Model file for the job. Use its own axes, mm. A direction names the side the tool comes from. Round coordinates to 2 decimals unless told otherwise and drop trailing zeros. Order: outer loops, then holes, each group sorted by start corner. A loop starts at its lowest first (then second) coordinate and runs counter-clockwise, first axis right, second up. Notation, with made-up numbers: (65.5, 76.5) -> (104.5, 76.5) arc R32 cw to (104.5, 105.5) -> close; hole circle Ø1 at (-38.5, 16.25). An arc over 180 degrees is marked (long way). Answer as CSV lines item,"result".
```python
from build123d import *

# Parameters (mm, degrees)
F0_R     = 7.5
F1_DEPTH = 20
F2_DEPTH = 35
F3_R     = 15
F4_DEPTH = 25
F5_R     = 3.175
F6_DEPTH = 31.5


with BuildPart() as f1:
    # F0 (on Top) → F1 (new body)
    with BuildSketch(Plane.XY):
        with BuildLine():
            Line((0, 40), (0, 50))
            ThreePointArc((0, 50), (-5.8547207654, 49.6560393584), (-11.6288897904, 48.6288897904))
            Line((-11.6288897904, 48.6288897904), (-5, 42))
            Line((-5, 42), (-15, 42))
            Line((-15, 42), (-15, 47.6969600708))
            ThreePointArc((-15, 47.6969600708), (-17.5249921621, 46.8281395073), (-20, 45.8257569496))
            Line((-20, 45.8257569496), (-20, -20))
            Line((-20, -20), (0, -20))
            Line((0, -20), (43.72135955, -20))
            Line((43.72135955, -20), (44.72135955, -20))
            Line((44.72135955, -20), (44.72135955, 1))
            ThreePointArc((44.72135955, 1), (44.4284663312, 0.2928932188), (43.72135955, 0))
            Line((43.72135955, 0), (40, 0))
            ThreePointArc((40, 0), (11.7157287525, 11.7157287525), (0, 40))
        make_face()
        with Locations((-10, -10)):
            Circle(F0_R, mode=Mode.SUBTRACT)
        Polygon((8, -5), (18, -5), (8, -15), align=None, mode=Mode.SUBTRACT)
        Polygon((35, -15), (25, -15), (35, -5), align=None, mode=Mode.SUBTRACT)
        Polygon((-15, 8), (-15, 18), (-5, 8), align=None, mode=Mode.SUBTRACT)
        Polygon((-5, 35), (-5, 25), (-15, 35), align=None, mode=Mode.SUBTRACT)
        with BuildLine():
            Line((0, 50), (0, 60))
            ThreePointArc((0, 60), (-10.1461187235, 59.1359135792), (-20, 56.5685424949))
            Line((-20, 56.5685424949), (-20, 45.8257569496))
            ThreePointArc((-20, 45.8257569496), (-17.5249921621, 46.8281395073), (-15, 47.6969600708))
            Line((-15, 47.6969600708), (-15, 52))
            Line((-15, 52), (-11.6288897904, 48.6288897904))
            ThreePointArc((-11.6288897904, 48.6288897904), (-5.8547207654, 49.6560393584), (0, 50))
        make_face()
        with BuildLine():
            Line((0, 60), (0, 70))
            ThreePointArc((0, 70), (-2.5032041292, 69.9552283185), (-5.0032061825, 69.8209705454))
            ThreePointArc((-5.0032061825, 69.8209705454), (-9.2928932188, 65.0502525317), (-14.7467938175, 68.4290294546))
            ThreePointArc((-14.7467938175, 68.4290294546), (-17.3864463232, 67.8064265704), (-20, 67.082039325))
            Line((-20, 67.082039325), (-20, 56.5685424949))
            ThreePointArc((-20, 56.5685424949), (-10.1461187235, 59.1359135792), (0, 60))
        make_face()
        with BuildLine():
            Line((0, 70), (0, 80))
            ThreePointArc((0, 80), (-10.0803433986, 79.3623757014), (-20, 77.4596669241))
            Line((-20, 77.4596669241), (-20, 67.082039325))
            ThreePointArc((-20, 67.082039325), (-17.3864463232, 67.8064265704), (-14.7467938175, 68.4290294546))
            ThreePointArc((-14.7467938175, 68.4290294546), (-10.7956226846, 74.936292591), (-5, 70))
            ThreePointArc((-5, 70), (-5.0008016099, 69.9104709192), (-5.0032061825, 69.8209705454))
            ThreePointArc((-5.0032061825, 69.8209705454), (-2.5032041292, 69.9552283185), (0, 70))
        make_face()
        with BuildLine():
            ThreePointArc((-20, 77.4596669241), (-10.0803433986, 79.3623757014), (0, 80))
            Line((0, 80), (-20, 80))
            Line((-20, 80), (-20, 77.4596669241))
        make_face()
        with BuildLine():
            ThreePointArc((50, 0), (48.6624494734, 11.4876460274), (44.72135955, 22.360679775))
            Line((44.72135955, 22.360679775), (44.72135955, 1))
            Line((44.72135955, 1), (44.72135955, -20))
            Line((44.72135955, -20), (44.72135955, -21))
            Line((44.72135955, -21), (44.72135955, -22.360679775))
            ThreePointArc((44.72135955, -22.360679775), (48.6624494734, -11.4876460274), (50, 0))
        make_face()
        with BuildLine():
            ThreePointArc((60, 0), (56.0503415378, 21.4093253864), (44.72135955, 40))
            Line((44.72135955, 40), (44.72135955, 22.360679775))
            ThreePointArc((44.72135955, 22.360679775), (48.6624494734, 11.4876460274), (50, 0))
            ThreePointArc((50, 0), (48.6624494734, -11.4876460274), (44.72135955, -22.360679775))
            Line((44.72135955, -22.360679775), (44.72135955, -40))
            ThreePointArc((44.72135955, -40), (56.0503415378, -21.4093253864), (60, 0))
        make_face()
        with BuildLine():
            ThreePointArc((70, 0), (66.7877004117, 20.9619434622), (57.4456264654, 40))
            Line((57.4456264654, 40), (44.72135955, 40))
            ThreePointArc((44.72135955, 40), (56.0503415378, 21.4093253864), (60, 0))
            ThreePointArc((60, 0), (56.0503415378, -21.4093253864), (44.72135955, -40))
            Line((44.72135955, -40), (57.4456264654, -40))
            ThreePointArc((57.4456264654, -40), (66.7877004117, -20.9619434622), (70, 0))
        make_face()
        with BuildLine():
            ThreePointArc((79.72135955, 6.6711941585), (76.3426815131, 23.9122349309), (69.2820323028, 40))
            Line((69.2820323028, 40), (57.4456264654, 40))
            ThreePointArc((57.4456264654, 40), (66.7877004117, 20.9619434622), (70, 0))
            ThreePointArc((70, 0), (66.7877004117, -20.9619434622), (57.4456264654, -40))
            Line((57.4456264654, -40), (69.2820323028, -40))
            ThreePointArc((69.2820323028, -40), (76.3426815131, -23.9122349309), (79.72135955, -6.6711941585))
            Line((79.72135955, -6.6711941585), (79.72135955, 6.6711941585))
        make_face()
        with BuildLine():
            ThreePointArc((69.2820323028, 40), (40, 69.2820323028), (0, 80))
            Line((0, 80), (0, 70))
            ThreePointArc((0, 70), (32.403703492, 62.04836823), (57.4456264654, 40))
            Line((57.4456264654, 40), (69.2820323028, 40))
        make_face()
        with BuildLine():
            ThreePointArc((44.72135955, 40), (24.4948974278, 54.7722557505), (0, 60))
            Line((0, 60), (0, 50))
            ThreePointArc((0, 50), (26.286555606, 42.5325404176), (44.72135955, 22.360679775))
            Line((44.72135955, 22.360679775), (44.72135955, 40))
        make_face()
        with BuildLine():
            Line((79.72135955, 40), (69.2820323028, 40))
            ThreePointArc((69.2820323028, 40), (76.3426815131, 23.9122349309), (79.72135955, 6.6711941585))
            Line((79.72135955, 6.6711941585), (79.72135955, 40))
        make_face()
        with BuildLine():
            ThreePointArc((79.72135955, -6.6711941585), (76.3426815131, -23.9122349309), (69.2820323028, -40))
            Line((69.2820323028, -40), (79.72135955, -40))
            Line((79.72135955, -40), (79.72135955, -6.6711941585))
        make_face()
    extrude(amount=F1_DEPTH)

    # F0 (on Top) → F2 (join)
    with BuildSketch(Plane.XY):
        with BuildLine():
            ThreePointArc((50, 0), (48.6624494734, 11.4876460274), (44.72135955, 22.360679775))
            Line((44.72135955, 22.360679775), (44.72135955, 1))
            Line((44.72135955, 1), (44.72135955, -20))
            Line((44.72135955, -20), (44.72135955, -21))
            Line((44.72135955, -21), (44.72135955, -22.360679775))
            ThreePointArc((44.72135955, -22.360679775), (48.6624494734, -11.4876460274), (50, 0))
        make_face()
        with BuildLine():
            ThreePointArc((60, 0), (56.0503415378, 21.4093253864), (44.72135955, 40))
            Line((44.72135955, 40), (44.72135955, 22.360679775))
            ThreePointArc((44.72135955, 22.360679775), (48.6624494734, 11.4876460274), (50, 0))
            ThreePointArc((50, 0), (48.6624494734, -11.4876460274), (44.72135955, -22.360679775))
            Line((44.72135955, -22.360679775), (44.72135955, -40))
            ThreePointArc((44.72135955, -40), (56.0503415378, -21.4093253864), (60, 0))
        make_face()
        with BuildLine():
            ThreePointArc((70, 0), (66.7877004117, 20.9619434622), (57.4456264654, 40))
            Line((57.4456264654, 40), (44.72135955, 40))
            ThreePointArc((44.72135955, 40), (56.0503415378, 21.4093253864), (60, 0))
            ThreePointArc((60, 0), (56.0503415378, -21.4093253864), (44.72135955, -40))
            Line((44.72135955, -40), (57.4456264654, -40))
            ThreePointArc((57.4456264654, -40), (66.7877004117, -20.9619434622), (70, 0))
        make_face()
        with BuildLine():
            ThreePointArc((79.72135955, 6.6711941585), (76.3426815131, 23.9122349309), (69.2820323028, 40))
            Line((69.2820323028, 40), (57.4456264654, 40))
            ThreePointArc((57.4456264654, 40), (66.7877004117, 20.9619434622), (70, 0))
            ThreePointArc((70, 0), (66.7877004117, -20.9619434622), (57.4456264654, -40))
            Line((57.4456264654, -40), (69.2820323028, -40))
            ThreePointArc((69.2820323028, -40), (76.3426815131, -23.9122349309), (79.72135955, -6.6711941585))
            Line((79.72135955, -6.6711941585), (79.72135955, 6.6711941585))
        make_face()
        with BuildLine():
            ThreePointArc((79.72135955, -6.6711941585), (76.3426815131, -23.9122349309), (69.2820323028, -40))
            Line((69.2820323028, -40), (79.72135955, -40))
            Line((79.72135955, -40), (79.72135955, -6.6711941585))
        make_face()
        with BuildLine():
            Line((79.72135955, 40), (69.2820323028, 40))
            ThreePointArc((69.2820323028, 40), (76.3426815131, 23.9122349309), (79.72135955, 6.6711941585))
            Line((79.72135955, 6.6711941585), (79.72135955, 40))
        make_face()
    extrude(amount=F2_DEPTH)

    # F3 (on face) → F4 (cut)
    with BuildSketch(Plane.YZ.offset(79.72135955)):
        with Locations((0, 17.5)):
            Circle(F3_R)
    extrude(amount=-F4_DEPTH, mode=Mode.SUBTRACT)

    # F5 (on face) → F6 (cut)
    with BuildSketch(Plane.XY.offset(35)):
        with Locations((72.72135955, 0)):
            Circle(F5_R)
    extrude(amount=-F6_DEPTH, mode=Mode.SUBTRACT)


solid = f1.part
```
Q1. Saw through at C-C (z = 30.5). Write the cut outline in (x, y).
Checks:
outline,"(44.72, -40) -> (79.72, -40) -> (79.72, -7.48) -> (54.72, -7.48) -> (54.72, 7.48) -> (79.72, 7.48) -> (79.72, 40) -> (44.72, 40) -> close"
Q2. Mould opens along X. For faces 4 (the flat face through (12, -20, 10)), 5 (the flat face through (-20, 31, 10)), 6 (the flat face through (0, 45, 10)) say: +X half, -X half, draft (parallel to the pull), parting line (faces both ways), or undercut.
Checks:
face 4,"draft"
face 5,"-X half"
face 6,"undercut"
Q3. Wall check: L1, parallel to Y at x = 71, z = 17; L2, parallel to Y at x = 3, z = 9; L3, parallel to X at y = 30, z = 7. Give the ranges that are in metal, low to high. Write a range as [from, to].
Checks:
L1,"[-40, -14.99], [14.99, 40]"
L2,"[-20, 24.8], [49.91, 59.92], [69.94, 79.94]"
L3,"[-20, -10], [-5, 1.27], [40, 79.72]"
Q4. Flat gauge pins, fed straight in: pin 1 (12 mm diameter, centred on x = 1.5, y = 47, fed in from -Z); pin 2 (4 mm diameter, centred on x = 5.5, z = 8, fed in from +Y); pin 3 (10 mm diameter, centred on x = 20, z = 7.5, fed in from -Y); pin 4 (3 mm diameter, centred on x = 28.5, z = 11.5, fed in from +Y). Where does each tip first touch, or does it go through?
Checks:
pin 1,"z = 0"
pin 2,"y = 79.92"
pin 3,"y = -20"
pin 4,"y = 75.31"
Q5. Saw through at A-A (x = -10). Write the cut outline in (y, z).
Checks:
outline,"(-20, 0) -> (-17.5, 0) -> (-17.5, 20) -> (-20, 20) -> close; (-2.5, 0) -> (8, 0) -> (8, 20) -> (-2.5, 20) -> close; (13, 0) -> (30, 0) -> (30, 20) -> (13, 20) -> close; (35, 0) -> (42, 0) -> (42, 20) -> (35, 20) -> close; (47, 0) -> (65, 0) -> (65, 20) -> (47, 20) -> close; (75, 0) -> (80, 0) -> (80, 20) -> (75, 20) -> close"
Q6. Tool access for faces 1 (the cylindrical face through (24.817, 54.627, 9.86)), 2 (the flat face through (44.721, 1, 21)), 3 (the flat face through (62, -40, 17)): list every direction of +Z, -Z, +X, -X, +Y, -Y with a clear straight run to the whole face (end or side of a thin tool).
Checks:
face 1,"+Z, -Z"
face 2,"+Z"
face 3,"+Z, -Z, +X, -X, -Y"
Q7. Saw through at D-D (y = 54). Write the cut outline in (x, z).
Checks:
outline,"(-20, 0) -> (26.15, 0) -> (26.15, 20) -> (-20, 20) -> close; (44.54, 0) -> (59.03, 0) -> (59.03, 20) -> (44.54, 20) -> close"
Q8. Saw through at B-B (y = 72). Write the cut outline in (x, z), plus the area to 3 significant figures.
Checks:
outline,"(-20, 0) -> (-14.58, 0) -> (-14.58, 20) -> (-20, 20) -> close; (-5.42, 0) -> (34.87, 0) -> (34.87, 20) -> (-5.42, 20) -> close"
area,"914 mm²"
